from build123d import *

# Parameters (mm, degrees)
SKETCH2_R           = 35
BOSS_EXTRUDE1_DEPTH = 6
SKETCH3_R           = 0.8
CUT_EXTRUDE1_DEPTH  = 6
SKETCH4_R           = 0.6
CUT_EXTRUDE2_DEPTH  = 6
SKETCH5_W           = 3
SKETCH5_H           = 10
BOSS_EXTRUDE2_DEPTH = 10
CUT_EXTRUDE3_DEPTH  = 55.790510127
SKETCH7_R           = 1.5
CUT_EXTRUDE4_DEPTH  = 55.790510127


with BuildPart() as part:
    # Sketch2 → Boss-Extrude1 (new body)
    with BuildSketch(Plane.XY):
        Circle(SKETCH2_R)
    extrude(amount=BOSS_EXTRUDE1_DEPTH)

    # Sketch3 → Cut-Extrude1 (cut)
    with BuildSketch(Plane.XY.offset(6)):
        with Locations((0, 30.914278185)):
            Circle(SKETCH3_R)
        with Locations((26.846787517, -15.585721815)):
            Circle(SKETCH3_R)
        with Locations((-26.846787517, -15.585721815)):
            Circle(SKETCH3_R)
    extrude(amount=-CUT_EXTRUDE1_DEPTH, mode=Mode.SUBTRACT)

    # Sketch4 → Cut-Extrude2 (cut)
    with BuildSketch(Plane.XY.offset(6)):
        Circle(SKETCH4_R)
    extrude(amount=-CUT_EXTRUDE2_DEPTH, mode=Mode.SUBTRACT)

    # Sketch5 → Boss-Extrude2 (add)
    with BuildSketch(Plane.XY.offset(6)):
        with Locations((2.5, 0)):
            Rectangle(SKETCH5_W, SKETCH5_H)
        with Locations((-2.5, 0)):
            Rectangle(SKETCH5_W, SKETCH5_H)
    extrude(amount=BOSS_EXTRUDE2_DEPTH)

    # Sketch6 → Cut-Extrude3 (cut, through all)
    with BuildSketch(Plane(origin=(4, 0, 0), x_dir=(0, 0, -1), z_dir=(1, 0, 0))):
        with BuildLine():
            ThreePointArc((-16, 0), (-14.535533906, 3.535533906), (-11, 5))
            Line((-11, 5), (-16, 5))
            Line((-16, 5), (-16, 0))
        make_face()
        with BuildLine():
            ThreePointArc((-11, -5), (-14.535533906, -3.535533906), (-16, 0))
            Line((-16, 0), (-16, -5))
            Line((-16, -5), (-11, -5))
        make_face()
    extrude(amount=-CUT_EXTRUDE3_DEPTH, mode=Mode.SUBTRACT)

    # Sketch7 → Cut-Extrude4 (cut, through all)
    with BuildSketch(Plane(origin=(4, 0, 0), x_dir=(0, 0, -1), z_dir=(1, 0, 0))):
        with Locations(Location((-11, 2.8, 0), (0, 0, 90))):
            Circle(SKETCH7_R)
        with Locations(Location((-11, -2.8, 0), (0, 0, 90))):
            Circle(SKETCH7_R)
    extrude(amount=-CUT_EXTRUDE4_DEPTH, mode=Mode.SUBTRACT)


solid = part.part
Input: part model. Units: mm. Frame: model coordinates. A direction names the side the tool comes from. Give positions to 0.01 mm unless a question says otherwise; leave off trailing zeros. Loops run counter-clockwise (first coordinate to the right, second up) from the corner with the lowest first, then second, coordinate; pieces in that order, holes last. Notation, with made-up numbers: (40, 70) -> (98, 70) arc R24 ccw to (98, 80) -> close; hole circle Ø1 at (61.5, -8.5). An arc over 180 degrees is marked (long way). Answer as a JSON object with one key per item and string values. Group by question number.
Item 1: Pull-direction query (Y, two-part tool) for faces 1 (the cylindrical face through (-2.48, -4.3, 11.07)), 2 (the flat face through (-3, -5, 8)), 3 (the flat face through (-4, 0, 11)); classes: released by +Y, released by -Y, zero draft, split by the parting line, or undercut.
Item 2: Line query: probe 1 along Y at (x, z) = (0, 2); probe 2 along Z at (x, y) = (-4.5, 21); probe 3 along Z at (x, y) = (-1.85, -2.8). Output: solid intervals per line, ascending.
Item 3: Reachability of faces 4 (the flat face through (-1, 0, 11)), 5 (the flat face through (2, -5, 8)), 6 (the flat face through (-3, 5, 8)), 7 (the flat face through (4, 0, 11)) from +Z, -Z, +X, -X, +Y, -Y: full face, straight path, thin tool, end or side. Return the list, or none.
Item 4: Cut plane C-C, the plane z = 2.5. Return the cut outline in (x, y), and give its area (3 significant figures).
Item 5: Cut plane B-B, the plane y = 2.8. Return the cut outline in (x, z), and give its area (3 significant figures).
Item 6: Cut plane D-D, the plane x = -10.5. Return the cut outline in (y, z).
Item 7: Pin query (flat end, axial travel): P1, Ø10, axis at x = -20.5, y = 24.5, coming from the +Z side; P2, Ø5, axis at y = 1, z = 13, coming from the +X side; P3, Ø2.5, axis at y = 2.8, z = 11, coming from the +X side; P4, Ø3.5, axis at x = 2.5, z = 8.5, coming from the +Y side. Return the tip coordinate at first contact, or that it passes through.
Item 8: Cut plane A-A, the plane z = 13.75. Return the cut outline in (x, y).
Checks:
{
 "1": {"face 1": "undercut", "face 2": "released by -Y", "face 3": "zero draft"},
 "2": {"probe 1": "y = -35 to -0.6, 0.6 to 30.11, 31.71 to 35", "probe 2": "z = 0 to 6", "probe 3": "z = 0 to 9.5, 12.5 to 15.14"},
 "3": {"face 4": "+Z, +Y, -Y", "face 5": "+Z, +X, -X, -Y", "face 6": "+Z, +X, -X, +Y", "face 7": "+Z, +X, +Y, -Y"},
 "4": {"outline": "circle Ø70 at (0, 0); hole circle Ø1.6 at (-26.85, -15.59); hole circle Ø1.6 at (0, 30.91); hole circle Ø1.2 at (0, 0); hole circle Ø1.6 at (26.85, -15.59)", "area": "3,840 mm²"},
 "5": {"outline": "(-34.89, 0) -> (34.89, 0) -> (34.89, 6) -> (4, 6) -> (4, 9.5) -> (1, 9.5) -> (1, 6) -> (-1, 6) -> (-1, 9.5) -> (-4, 9.5) -> (-4, 6) -> (-34.89, 6) -> close; (-4, 12.5) -> (-1, 12.5) -> (-1, 15.14) -> (-4, 15.14) -> close; (1, 12.5) -> (4, 12.5) -> (4, 15.14) -> (1, 15.14) -> close", "area": "456 mm²"},
 "6": {"outline": "(-33.39, 0) -> (33.39, 0) -> (33.39, 6) -> (-33.39, 6) -> close"},
 "7": {"P1": "stops at z = 6", "P2": "stops at x = 4", "P3": "passes through", "P4": "stops at y = 5"},
 "8": {"outline": "(-4, -4.18) -> (-1, -4.18) -> (-1, 4.18) -> (-4, 4.18) -> close; (1, -4.18) -> (4, -4.18) -> (4, 4.18) -> (1, 4.18) -> close"}
}
